The drawing under review shows one solid part. Ordinate dimensions are in mm from its lowest x, y, z. A direction names the side the tool comes from. Round coordinates to 2 decimals unless told otherwise and drop trailing zeros. Write each loop counter-clockwise with the first axis right and the second up, starting at its lowest first coordinate (ties: lowest second). Pieces come first, ordered by that corner, then holes. Notation, with made-up numbers: (56, -0.75) -> (65, -0.75) arc R16 ccw to (65, 5.25) -> close; hole circle Ø10 at (63.5, -31.5). An arc over 180 degrees is marked (long way). Write item = value, one per line. Start each with the question number.
Item 1: For pin 1 Ø4 at (x, y) = (5.5, 5.5) entering from -Z; pin 2 Ø3 at (x, z) = (9.5, 14.5) entering from +Y; pin 3 Ø1 at (y, z) = (3.5, 6) entering from +X, all flat-tipped, find the tip position at first contact; note any pin that passes through.
Item 2: Add section C-C, the plane z = 4.75. State the section outline as (x, y) points, then the cut area to 3 significant figures.
Item 3: Add section D-D, the plane y = 8.5. State the section outline as (x, z) points, then the cut area to 3 significant figures.
Item 4: Machinability: for the marked faces 4 and 5, which of the approach directions +Z, -Z, +X, -X, +Y, -Y give a long, thin tool a straight path to every point of the face, cutting with its end or side? Answer none if there is none.
Item 5: To check wall thickness, follow L1, parallel to Y at x = 5.5, z = 2; L2, parallel to Y at x = 5.5, z = 3.7; L3, parallel to Z at x = 4, y = 2.75. State the ranges of each line that lie inside material, in increasing order.
Item 6: Add section A-A, the plane y = 5.25. State the section outline as (x, z) points, then the cut area to 3 significant figures.
Item 7: Add section B-B, the plane x = 5.5. State the section outline as (y, z) points.
Item 8: Mouldability with a two-part tool opening along Y and no side actions: class the marked faces 1, 2 and 3 as released by +Y, released by -Y, zero draft, split by the parting line, or undercut.
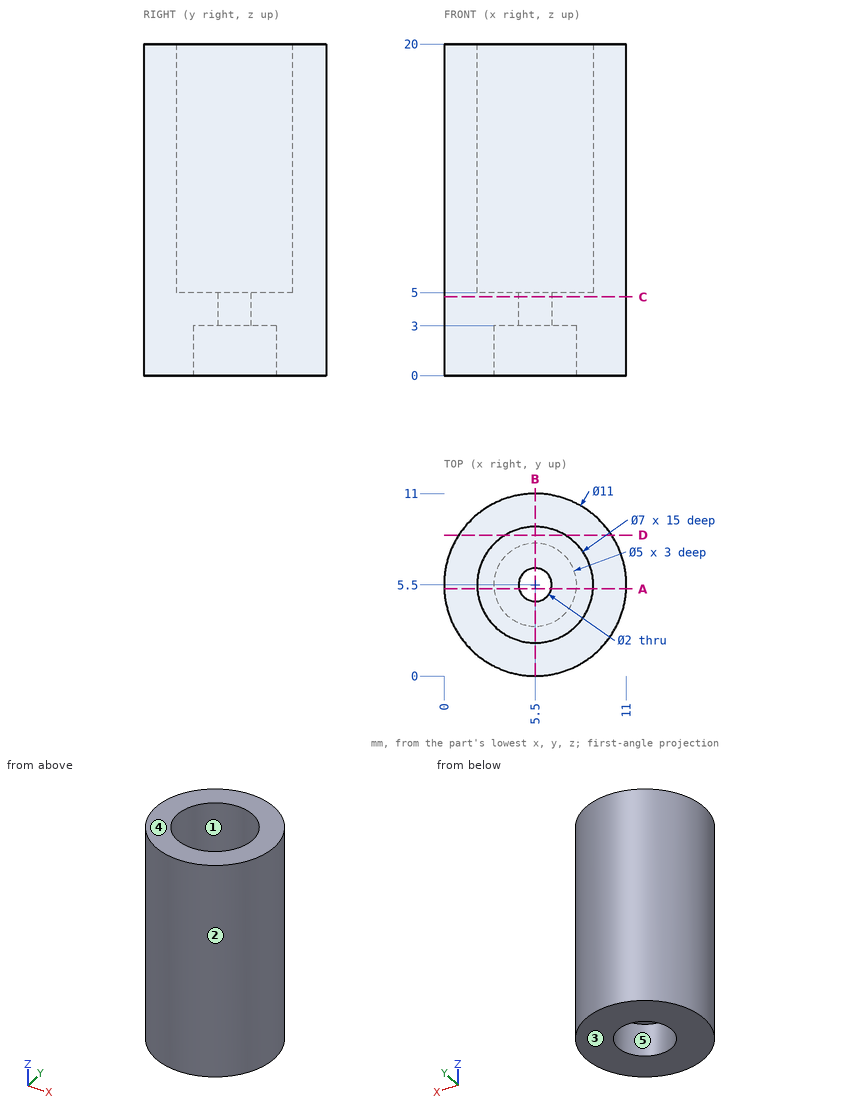
Result set:
q1.pin_1 = 3
q1.pin_2 = 10.4
q1.pin_3 = 10.79
q2.outline = circle Ø11 at (5.5, 5.5); hole circle Ø2 at (5.5, 5.5)
q2.area = 91.9 mm²
q3.outline = (0.89, 0) -> (10.11, 0) -> (10.11, 20) -> (7.3, 20) -> (7.3, 5) -> (3.7, 5) -> (3.7, 20) -> (0.89, 20) -> close
q3.area = 130 mm²
q4.face_4 = +Z, +X, -X, +Y, -Y
q4.face_5 = -Z
q5.L1 = 0 to 3, 8 to 11
q5.L2 = 0 to 4.5, 6.5 to 11
q5.L3 = 0 to 5
q6.outline = (0.01, 0) -> (3.01, 0) -> (3.01, 3) -> (4.53, 3) -> (4.53, 5) -> (2.01, 5) -> (2.01, 20) -> (0.01, 20) -> close; (6.47, 3) -> (7.99, 3) -> (7.99, 0) -> (10.99, 0) -> (10.99, 20) -> (8.99, 20) -> (8.99, 5) -> (6.47, 5) -> close
q6.area = 96.2 mm²
q7.outline = (0, 0) -> (3, 0) -> (3, 3) -> (4.5, 3) -> (4.5, 5) -> (2, 5) -> (2, 20) -> (0, 20) -> close; (6.5, 3) -> (8, 3) -> (8, 0) -> (11, 0) -> (11, 20) -> (9, 20) -> (9, 5) -> (6.5, 5) -> close
q8.face_1 = undercut
q8.face_2 = split by the parting line
q8.face_3 = zero draft
